from build123d import *

# Parameters (mm, degrees)
F1_DEPTH = 2.5
F2_DEPTH = 1.25
F0_R     = 2.5
F3_DEPTH = 2.5
F4_DEPTH = 2.5


with BuildPart() as f1:
    # F0 (on Right) → F1 (new body, symmetric)
    with BuildSketch(Plane.YZ):
        with BuildLine():
            ThreePointArc((152.05, -2.5), (155.212278, -3.013167), (158.05, -4.5))
            Line((158.05, -4.5), (152.05, 0))
            Line((152.05, 0), (-152.05, 0))
            Line((-152.05, 0), (-158.05, -4.5))
            ThreePointArc((-158.05, -4.5), (-155.212278, -3.013167), (-152.05, -2.5))
            Line((-152.05, -2.5), (152.05, -2.5))
        make_face()
    extrude(amount=F1_DEPTH, both=True)



with BuildPart() as f2:
    # F0 (on Right) → F2 (new body, symmetric)
    with BuildSketch(Plane.YZ):
        with BuildLine():
            Line((-142.05, -12.5), (142.05, -12.5))
            ThreePointArc((142.05, -12.5), (144.978932, -5.428932), (152.05, -2.5))
            Line((152.05, -2.5), (-152.05, -2.5))
            ThreePointArc((-152.05, -2.5), (-144.978932, -5.428932), (-142.05, -12.5))
        make_face()
    extrude(amount=F2_DEPTH, both=True)


with BuildPart() as f1_1:
    add(f1.part)

    add(f2.part)  # F3 merges F2
    # F0 (on Right) → F3 (join)
    with BuildSketch(Plane.YZ):
        with BuildLine():
            ThreePointArc((-158.05, -4.5), (-156.522136, -21.444272), (-142.05, -12.5))
            ThreePointArc((-142.05, -12.5), (-144.978932, -5.428932), (-152.05, -2.5))
            ThreePointArc((-152.05, -2.5), (-155.212278, -3.013167), (-158.05, -4.5))
        make_face()
        with Locations((-152.05, -12.5)):
            Circle(F0_R, mode=Mode.SUBTRACT)
    extrude(amount=F3_DEPTH)

    # F0 (on Right) → F4 (join)
    with BuildSketch(Plane.YZ):
        with BuildLine():
            ThreePointArc((142.05, -12.5), (152.05, -22.5), (162.05, -12.5))
            ThreePointArc((162.05, -12.5), (160.994272, -8.027864), (158.05, -4.5))
            ThreePointArc((158.05, -4.5), (155.212278, -3.013167), (152.05, -2.5))
            ThreePointArc((152.05, -2.5), (144.978932, -5.428932), (142.05, -12.5))
        make_face()
        with Locations((152.05, -12.5)):
            Circle(F0_R, mode=Mode.SUBTRACT)
    extrude(amount=-F4_DEPTH)


solid = f1_1.part
Input: part model. Units: mm. Frame: model coordinates. Give positions to 0.01 mm unless a question says otherwise; leave off trailing zeros. Order: outer loops, then holes, each group sorted by start corner. A loop starts at its lowest first (then second) coordinate and runs counter-clockwise, first axis right, second up.
Q1. Contact query for flat-ended pins moving along their axis: pin 1 Ø8 at (y, z) = (-114, -8.5) entering from -X; pin 2 Ø1 at (x, y) = (2, 31.5) entering from -Z; pin 3 Ø3 at (x, y) = (1.5, -42) entering from +Z; pin 4 Ø2 at (x, z) = (-0.5, -3) entering from -Y. Output: stop coordinate, or through.
Checked values:
pin 1: stops at x = -1.25
pin 2: stops at z = -2.5
pin 3: stops at z = 0
pin 4: stops at y = -157.38
Q2. Draft query along Y for faces 1 (the cylindrical face through (1.23, -149.74, -13.46)), 2 (the flat face through (2.5, -50, -2)), 3 (the flat face through (0.04, 155.09, -2.28)). Return one class per face: +Y half, -Y half, draft (parallel to the pull), parting line (faces both ways), or undercut.
Checked values:
face 1: undercut
face 2: draft
face 3: +Y half
Q3. Ray query, probe 1 along Z at (x, y) = (0.85, -152.05); probe 2 along Z at (x, y) = (-1.45, 46); probe 3 along X at (y, z) = (48, -3). Return the intervals inside material, ascending.
Checked values:
probe 1: z = -22.5 to -15, -10 to 0
probe 2: z = -2.5 to 0
probe 3: x = -1.25 to 1.25
Q4. Section A-A on y = 37. Output: boundary loops of the cut face in (x, z), and give its area (3 significant figures).
Checked values:
outline: (-2.5, -2.5) - (-1.25, -2.5) - (-1.25, -12.5) - (1.25, -12.5) - (1.25, -2.5) - (2.5, -2.5) - (2.5, 0) - (-2.5, 0) - close
area: 37.5 mm2
